```python
from build123d import *

# Parameters (mm, degrees)
BOSS_EXTRUDE1_DEPTH = 2
FILLET1_R           = 0.25
SKETCH3_W           = 26
SKETCH3_H           = 12
CUT_EXTRUDE2_DEPTH  = 1
FILLET6_R           = 2


with BuildPart() as part:
    # Sketch1 → Boss-Extrude1 (new body)
    with BuildSketch(Plane(origin=(0, 0, 0), x_dir=(1, 0, 0), z_dir=(0, 1, 0))):
        Polygon((-15, 2.618365096), (-20, 3.5), (-20, -3.5), (-15, -2.618365096), (-15, -6), (15, -6), (15, -2.618365096), (20, -3.5), (20, 3.5), (15, 2.618365096), (15, 6), (-15, 6), align=None)
    extrude(amount=BOSS_EXTRUDE1_DEPTH)

    # Fillet1
    fillet1_edges = [part.edges().sort_by_distance(p)[0] for p in [
        (15, 1, -2.618365096),
        (20, 1, -3.5),
        (20, 1, 3.5),
        (15, 1, 2.618365096),
        (-15, 1, 2.618365096),
        (-20, 1, 3.5),
        (-20, 1, -3.5),
        (-15, 1, -2.618365096),
    ]]
    fillet(fillet1_edges, radius=FILLET1_R)

    # Sketch3 → Cut-Extrude2 (cut)
    with BuildSketch(Plane(origin=(0, 2, 0), x_dir=(1, 0, 0), z_dir=(0, 1, 0))):
        Rectangle(SKETCH3_W, SKETCH3_H)
    extrude(amount=-CUT_EXTRUDE2_DEPTH, mode=Mode.SUBTRACT)

    # Fillet6
    # the kernel refuses this fillet: 2 mm, written as the material it adds along each edge
    with BuildSketch(Plane(origin=(-13, 1, 6), x_dir=(0, 1, 0), z_dir=(0, 0, -1))) as fillet6_piece_1:
        with BuildLine():
            CenterArc((2, 1.732050808), FILLET6_R, 180, 60)
            Line((0, 1.732050808), (-0.04, 1.732050808))
            Line((-0.04, 1.732050808), (-0.04, 0))
            Line((-0.04, 0), (0, -0.04))
            ThreePointArc((0, -0.04), (0.5, -0.04), (0.98, -0.034641016))
            Line((0.98, -0.034641016), (1, 0))
        make_face()
    extrude(amount=12)
    with BuildSketch(Plane(origin=(13, 1, -6), x_dir=(-1, 0, 0), z_dir=(0, 0, 1))) as fillet6_piece_2:
        with BuildLine():
            CenterArc((1.732050808, -2), FILLET6_R, 90, 60)
            Line((0, -1), (-0.034641016, -0.98))
            ThreePointArc((-0.034641016, -0.98), (-0.04, -0.5), (-0.04, 0))
            Line((-0.04, 0), (0, 0.04))
            Line((0, 0.04), (1.732050808, 0.04))
            Line((1.732050808, 0.04), (1.732050808, 0))
        make_face()
    extrude(amount=12)


solid = part.part
```
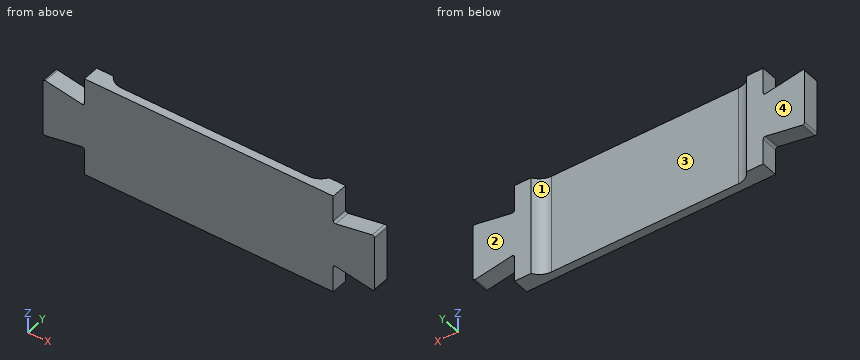
The listing builds one solid part. Answer for the finished solid, in the listing's coordinates (mm). Face numbers are marked on the shaded views. A direction names the side the tool comes from. Round coordinates to 2 decimals unless told otherwise and drop trailing zeros. Loops run counter-clockwise (first coordinate to the right, second up) from the corner with the lowest first, then second, coordinate; pieces in that order, holes last. Notation, with made-up numbers: (30.5, 72) - (68.5, 72) arc R18 ccw to (68.5, 100) - close; hole circle Ø2 at (1, 70). An arc over 180 degrees is marked (long way). Return JSON: item names as keys, results as strings. Group by question number.
1. Consider probe 1 along Y at (x, z) = (10, -5); probe 2 along X at (y, z) = (0.9, -5); probe 3 along X at (y, z) = (1.6, -2.5). Determine where each line is inside the solid, lowest interval first.
2. The part is cut by section A-A on z = -1.75. Determine the outline of the cut face in (x, y), then the cut area to 3 significant figures.
3. Each of these flat-tipped pins is pushed along its axis until it touches: P1, Ø6, axis at x = 4.5, z = 2.5, coming from the +Y side; P2, Ø1, axis at y = 0.5, z = -5, coming from the +X side. Where does it stop, or does it pass through?
4. The part is cut by section C-C on z = 4.5. Determine the outline of the cut face in (x, y).
5. Which of the six approach directions +Z, -Z, +X, -X, +Y, -Y give full straight-line access (tool end or side, diameter ignored) to the marked faces 3 and 4?
6. The part is cut by section D-D on x = 12. Determine the outline of the cut face in (y, z), then the cut area to 3 significant figures.
7. The mould has two halves that part along X. Classify the marked faces 1 and 2: pulls with the +X half, pulls with the -X half, needs draft (parallel to the pull), parting line crosses it, or undercut.
8. The part is cut by section B-B on y = 0.4. Determine the outline of the cut face in (x, z).
Resolved:
{
 "1": {"probe 1": "y = 0 to 1", "probe 2": "x = -15 to 15", "probe 3": "x = -20 to -12.7, 12.7 to 20"},
 "2": {"outline": "(-20, 0) - (20, 0) - (20, 2) - (13, 2) arc R2 cw to (11.27, 1) - (-11.27, 1) arc R2 cw to (-13, 2) - (-20, 2) - close", "area": "55.0 mm²"},
 "3": {"P1": "stops at y = 1", "P2": "stops at x = 15"},
 "4": {"outline": "(-15, 0) - (15, 0) - (15, 2) - (13, 2) arc R2 cw to (11.27, 1) - (-11.27, 1) arc R2 cw to (-13, 2) - (-15, 2) - close"},
 "5": {"face 3": "+Z, -Z, +Y", "face 4": "+Z, -Z, +X, -X, +Y"},
 "6": {"outline": "(0, -6) - (1.14, -6) - (1.14, 6) - (0, 6) - close", "area": "13.7 mm²"},
 "7": {"face 1": "undercut", "face 2": "needs draft"},
 "8": {"outline": "(-20, -3.2) arc R0.25 ccw to (-19.71, -3.45) - (-15.29, -2.67) arc R0.25 cw to (-15, -2.92) - (-15, -6) - (15, -6) - (15, -2.92) arc R0.25 cw to (15.29, -2.67) - (19.71, -3.45) arc R0.25 ccw to (20, -3.2) - (20, 3.2) arc R0.25 ccw to (19.71, 3.45) - (15.29, 2.67) arc R0.25 cw to (15, 2.92) - (15, 6) - (-15, 6) - (-15, 2.92) arc R0.25 cw to (-15.29, 2.67) - (-19.71, 3.45) arc R0.25 ccw to (-20, 3.2) - close"}
}
